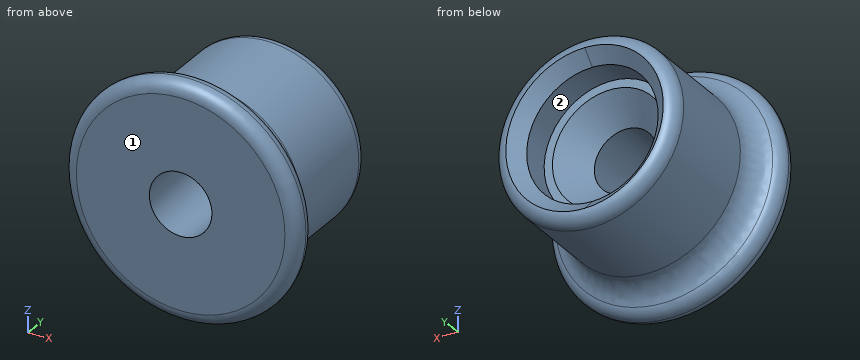
```python
from build123d import *

# Parameters (mm, degrees)
SKETCH4_R           = 5.55625
SKETCH4_R_2         = 1.905
BOSS_EXTRUDE3_DEPTH = 9.525
SKETCH5_R           = 7.14375
SKETCH5_R_2         = 1.905
BOSS_EXTRUDE4_DEPTH = 1.5875
FILLET4_R           = 0.79375
FILLET5_R           = 1.5875
SKETCH6_R           = 4.0005
CUT_EXTRUDE1_DEPTH  = 2.54
CHAMFER1_SIZE       = 0.79375
CHAMFER2_SIZE       = 1.5875


with BuildPart() as part:
    # Sketch4 → Boss-Extrude3 (new body)
    with BuildSketch(Plane(origin=(0, 0, 0), x_dir=(1, 0, 0), z_dir=(0, 1, 0))):
        with Locations(Location((0, 0, 0), (0, 0, 90))):
            Circle(SKETCH4_R)
        with Locations(Location((0, 0, 0), (0, 0, 90))):
            Circle(SKETCH4_R_2, mode=Mode.SUBTRACT)
    extrude(amount=BOSS_EXTRUDE3_DEPTH)

    # Sketch5 → Boss-Extrude4 (add)
    with BuildSketch(Plane(origin=(0, 0, 0), x_dir=(-1, 0, 0), z_dir=(0, -1, 0))):
        with Locations(Location((0, 0, 0), (0, 0, 90))):
            Circle(SKETCH5_R)
        with Locations(Location((0, 0, 0), (0, 0, 90))):
            Circle(SKETCH5_R_2, mode=Mode.SUBTRACT)
    extrude(amount=-BOSS_EXTRUDE4_DEPTH)

    # Fillet4
    fillet4_edges = [part.edges().sort_by_distance(p)[0] for p in [
        (0, 0, 7.14375),
        (0, 1.5875, 7.14375),
        (0, 9.525, 5.55625),
    ]]
    fillet(fillet4_edges, radius=FILLET4_R - 0.0001)  # a hair under: the kernel refuses the full size

    # Fillet5
    fillet5_edges = [part.edges().sort_by_distance(p)[0] for p in [
        (0, 1.5875, 5.55625),
    ]]
    fillet(fillet5_edges, radius=FILLET5_R)

    # Sketch6 → Cut-Extrude1 (cut)
    with BuildSketch(Plane(origin=(0, 9.525, 0), x_dir=(1, 0, 0), z_dir=(0, 1, 0))):
        with Locations(Location((0, 0, 0), (0, 0, 270))):
            Circle(SKETCH6_R)
    extrude(amount=-CUT_EXTRUDE1_DEPTH, mode=Mode.SUBTRACT)

    # Chamfer1
    chamfer1_edges = [part.edges().sort_by_distance(p)[0] for p in [
        (0, 9.525, -4.0005),
    ]]
    chamfer(chamfer1_edges, length=CHAMFER1_SIZE)

    # Chamfer2
    chamfer2_edges = [part.edges().sort_by_distance(p)[0] for p in [
        (0, 6.985, 1.905),
    ]]
    chamfer(chamfer2_edges, length=CHAMFER2_SIZE)


solid = part.part
```
Part model, mm, in its own coordinate system. Face numbers are marked on the shaded views. A direction names the side the tool comes from. Coordinates: 2 decimals unless noted, no trailing zeros. Write each loop counter-clockwise with the first axis right and the second up, starting at its lowest first coordinate (ties: lowest second). Pieces come first, ordered by that corner, then holes.
Item 1: Pin check, flat tips, straight feed: pin 1 (5 mm diameter, centred on y = 6.5, z = 4.5, fed in from -X); pin 2 (2 mm diameter, centred on x = -2, y = 3.5, fed in from -Z); pin 3 (1.5 mm diameter, centred on y = 6, z = -2.5, fed in from -X). Stop position of each tip, or through.
Item 2: Slice it at A-A (y = 5). Write the cut outline in (x, z) (1 decimal).
Item 3: Slice it at B-B (y = 8). Write the cut outline in (x, z), and give its area (3 significant figures).
Item 4: Probe line 1 (X direction, y = 8.1, z = 0); line 2 (Z direction, x = -1.75, y = 4.5); line 3 (Z direction, x = -1.5, y = 9). List the from-to ranges inside material, lowest first.
Item 5: Which spindle directions (+Z, -Z, +X, -X, +Y, -Y) get a long thin tool onto all of the face, cutting with end or side? Do the marked faces 1 and 2. Say none if no direction does.
Results found:
1. pin 1: stops at x = -5.18
1. pin 2: stops at z = -5.47
1. pin 3: stops at x = -5.27
2. outline: circle Ø11.1 at (0, 0); hole circle Ø3.8 at (0, 0)
3. outline: circle Ø11.11 at (0, 0); hole circle Ø8 at (0, 0)
3. area: 46.7 mm2
4. line 1: x = -5.56 to -4, 4 to 5.56
4. line 2: z = -5.27 to -0.75, 0.75 to 5.27
4. line 3: z = -5.3 to -4, 4 to 5.3
5. face 1: +Z, -Z, +X, -X, -Y
5. face 2: +Y
